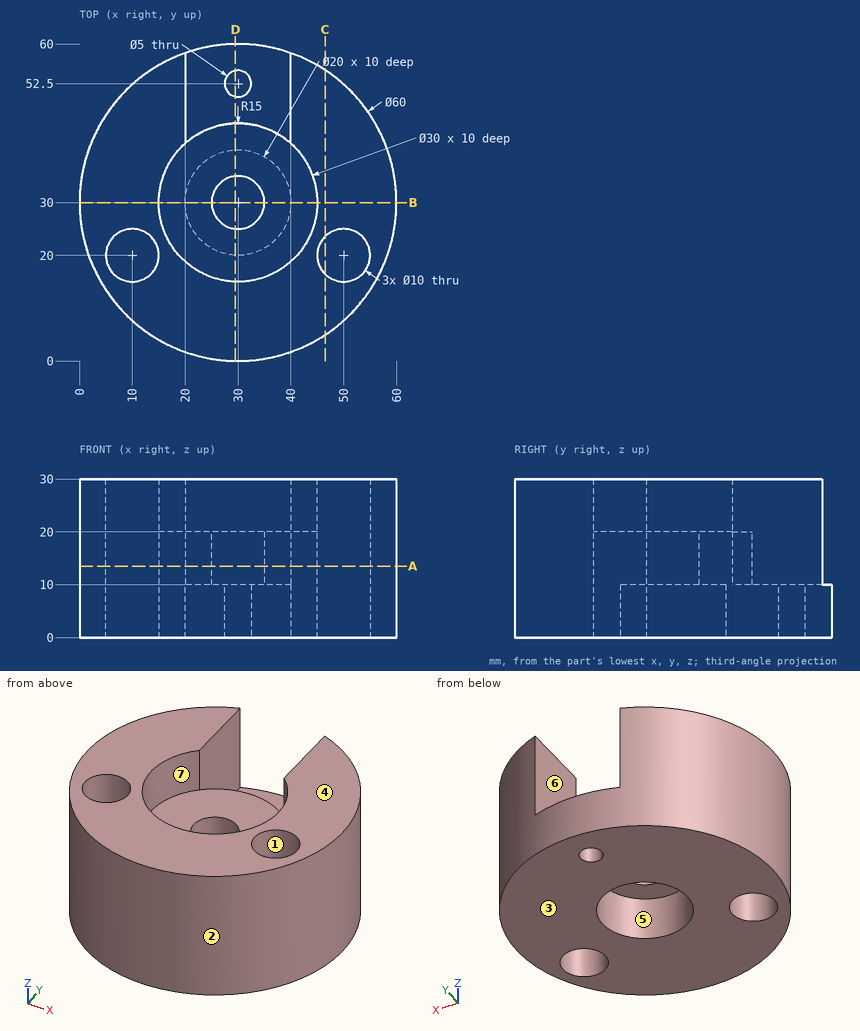
Input: dimensioned drawing with shaded views. Units: mm. Origin: part minimum x, y, z. A direction names the side the tool comes from. Coordinates: 2 decimals unless noted, no trailing zeros. Order: outer loops, then holes, each group sorted by start corner. A loop starts at its lowest first (then second) coordinate and runs counter-clockwise, first axis right, second up.
(1) Section query B-B (y = 30). Return the cut outline in (x, z), plus the area to 3 significant figures.
(2) Section query C-C (x = 46.5). Return the cut outline in (y, z).
(3) Material intervals for probe 1 along Y at (x, z) = (30, 17.25); probe 2 along X at (y, z) = (42, 11.5); probe 3 along Y at (x, z) = (30, 5.5), sorted ascending.
(4) Draft query along X for the marked faces 1, 2 and 3. Return one class per face: pulls with the +X half, pulls with the -X half, needs draft (parallel to the pull), parting line crosses it, or undercut.
(5) Section query D-D (x = 29.5). Return the cut outline in (y, z), plus the area to 3 significant figures.
(6) Section query A-A (z = 13.5). Return the cut outline in (x, y).
(7) First-contact query: pin 1 (6 mm diameter, centred on x = 17, z = 14.5, fed in from -Y); pin 2 (2 mm diameter, centred on y = 41.5, z = 12, fed in from -X); pin 3 (4 mm diameter, centred on x = 36.5, z = 21.5, fed in from +Y); pin 4 (16 mm diameter, centred on x = 10, y = 20, fed in from +Z). Flat tips, straight axial feed; report the tip coordinate or a pass-through.
(8) Access query for the marked faces 4, 5, 6 and 7. Directions: +Z, -Z, +X, -X, +Y, -Y. A direction counts if a zero-diameter tool reaches every point of the face in a straight line with its end or side. Return the directions, or none.
Solution:
1. outline: (0, 0) - (20, 0) - (20, 10) - (25, 10) - (25, 20) - (15, 20) - (15, 30) - (0, 30) - close; (35, 10) - (40, 10) - (40, 0) - (60, 0) - (60, 30) - (45, 30) - (45, 20) - (35, 20) - close
1. area: 1,200 mm2
2. outline: (4.95, 0) - (16.43, 0) - (16.43, 30) - (4.95, 30) - close; (23.57, 0) - (55.05, 0) - (55.05, 30) - (23.57, 30) - close
3. probe 1: y = 0 to 25, 35 to 45
3. probe 2: x = 2.5 to 20, 21 to 39, 40 to 57.5
3. probe 3: y = 0 to 20, 40 to 50, 55 to 60
4. face 1: undercut
4. face 2: parting line crosses it
4. face 3: needs draft
5. outline: (0, 0) - (20.01, 0) - (20.01, 10) - (25.03, 10) - (25.03, 20) - (15.01, 20) - (15.01, 30) - (0, 30) - close; (34.97, 10) - (39.99, 10) - (39.99, 0) - (50.05, 0) - (50.05, 10) - (44.99, 10) - (44.99, 20) - (34.97, 20) - close; (54.95, 0) - (60, 0) - (60, 10) - (54.95, 10) - close
5. area: 852 mm2
6. outline: (20, 41.18) - (20, 58.28) arc R30 ccw (long way) to (40, 58.28) - (40, 41.18) arc R15 ccw to start; hole circle Ø10 at (10, 20); hole circle Ø10 at (30, 30); hole circle Ø10 at (50, 20)
7. pin 1: stops at y = 1.72
7. pin 2: stops at x = 1.9
7. pin 3: stops at y = 44.08
7. pin 4: stops at z = 30
8. face 4: +Z, +X, -X, +Y, -Y
8. face 5: -Z
8. face 6: +Z, +Y
8. face 7: +Z
